Autodesk Inventor part; units mm, degrees
ref_plane "YZ Plane" through (0, 0, 0) normal (1, 0, 0) x (0, 1, 0)
ref_plane "XZ Plane" through (0, 0, 0) normal (0, 1, 0) x (-1, 0, 0)
ref_plane "XY Plane" through (0, 0, 0) normal (0, 0, 1) x (1, 0, 0)
sketch "Sketch1" plane through (0, 0, 0) normal (0, 0, 1) x (1, 0, 0)
  line L0 (-12.1708, 16.0073) -> (13.2292, 16.0073)
  line L1 (13.2292, 16.0073) -> (13.2292, -34.7927)
  line L2 (13.2292, -34.7927) -> (-12.1708, -34.7927)
  line L3 (-12.1708, -34.7927) -> (-12.1708, 16.0073)
  line L4 (11.9592, 14.7373) -> (-10.9008, 14.7373)
  line L5 (-10.9008, 14.7373) -> (-10.9008, -33.5227)
  line L6 (-10.9008, -33.5227) -> (11.9592, -33.5227)
  line L7 (11.9592, -33.5227) -> (11.9592, 14.7373)
  point P0 (0, 0)
  dimension "d0" = 25.4
  dimension "d1" = 50.8
  dimension "d2" = 1.27
extrude "Extrusion1" add sketch "Sketch1" along normal blind 76.2
sketch "Sketch2" plane through (-12.1708, 16.0073, 0) normal (0, 1, 0) x (1, 0, 0)
  circle A0 centre (12.7, -12.7) radius 1.7272
  line L0 (25.4, 0) -> (0, 0)
  line L1 (0, 0) -> (0, -76.2)
  point P0 (12.1708, 0)
  dimension "d5" = 3.4544
  dimension "d6" = 12.7
  dimension "d7" = 12.7
extrude "Extrusion2" cut sketch "Sketch2" against normal through all
pattern_linear "Rectangular Pattern1" count 8 spacing 25.4 along (0, 0, 1) of "Extrusion2"
sketch "Sketch3" plane through (13.2292, -34.7927, 0) normal (1, 0, 0) x (0, 0, -1)
  circle A0 centre (-38.1, 25.4) radius 14.2875
  line L0 (0, 0) -> (-76.2, 0)
  line L1 (-76.2, 0) -> (-76.2, 50.8)
  point P0 (0, 34.7927)
  dimension "d15" = 25.4
  dimension "d16" = 38.1
  dimension "d17" = 28.575
extrude "Extrusion3" cut sketch "Sketch3" against normal through all
equation "\"d3\" = d13"
equation "\"d10\" = d14"
equation "\"d13\" = 76.2"
equation "\"d14\" = d13"
properties part number "Test  Stock Rotation extender"
Input: part model. Units: mm. Frame: model coordinates. A direction names the side the tool comes from. Coordinates: 2 decimals unless noted, no trailing zeros. Order: outer loops, then holes, each group sorted by start corner. A loop starts at its lowest first (then second) coordinate and runs counter-clockwise, first axis right, second up. Notation, with made-up numbers: M -14.5,56.5 L 32.5,56.5 A12 ccw 32.5,60.5 Z; hole C 49,81 d11. An arc over 180 degrees is marked long. Write item = value, one per line. Start each with the question number.
(1) Section C-C on x = -2. Output: boundary loops of the cut face in (y, z).
(2) Section A-A on z = 12.7. Output: boundary loops of the cut face in (x, y).
(3) Section D-D on z = 38.1. Output: boundary loops of the cut face in (x, y), and give its area (3 significant figures).
(4) Pull-direction query (Z, two-part tool) for faces 3 (the flat face through (-10.901, 7, 38)), 4 (the cylindrical face through (0.3, -34.15, 10.99)), 5 (the flat face through (-12, -9, 0)), 6 (the cylindrical face through (12.603, -5.101, 24.472)); classes: released by +Z, released by -Z, zero draft, split by the parting line, or undercut.
(5) Section B-B on y = -28.5. Output: boundary loops of the cut face in (x, z).
(6) First-contact query: P1, Ø2, axis at x = 0.53, z = 12.7, coming from the +Y side. Flat tip, straight axial feed; report the tip coordinate or a pass-through.
(7) Line query: line 1 along X through (y, z) = (-33.95, 38.1); line 2 along Y through (x, z) = (-10.5, 13.5); line 3 along X through (y, z) = (-19.5, 17.5). Output: solid intervals per line, ascending. Write a range as [from, to].
(8) Reachability of faces 1 (the flat face through (4, -34.793, 38)), 2 (the flat face through (11.959, 6, 38)) from +Z, -Z, +X, -X, +Y, -Y: full face, straight path, thin tool, end or side. Return the list, or none.
Result set:
q1.outline = M -34.79,0 L -33.52,0 L -33.52,76.2 L -34.79,76.2 Z; M 14.74,0 L 16.01,0 L 16.01,76.2 L 14.74,76.2 Z
q2.outline = M -12.17,-34.79 L -1.2,-34.79 L -1.2,-33.52 L -10.9,-33.52 L -10.9,14.74 L -1.2,14.74 L -1.2,16.01 L -12.17,16.01 Z; M 2.26,-34.79 L 13.23,-34.79 L 13.23,16.01 L 2.26,16.01 L 2.26,14.74 L 11.96,14.74 L 11.96,-33.52 L 2.26,-33.52 Z
q3.outline = M -12.17,-34.79 L -1.2,-34.79 L -1.2,-33.52 L -10.9,-33.52 L -10.9,-23.68 L -12.17,-23.68 Z; M -12.17,4.89 L -10.9,4.89 L -10.9,14.74 L -1.2,14.74 L -1.2,16.01 L -12.17,16.01 Z; M 2.26,-34.79 L 13.23,-34.79 L 13.23,-23.68 L 11.96,-23.68 L 11.96,-33.52 L 2.26,-33.52 Z; M 2.26,14.74 L 11.96,14.74 L 11.96,4.89 L 13.23,4.89 L 13.23,16.01 L 2.26,16.01 Z
q3.area = 106 mm²
q4.face_3 = zero draft
q4.face_4 = undercut
q4.face_5 = released by -Z
q4.face_6 = undercut
q5.outline = M -12.17,0 L -10.9,0 L -10.9,76.2 L -12.17,76.2 Z; M 11.96,0 L 13.23,0 L 13.23,76.2 L 11.96,76.2 Z
q6.P1 = through
q7.line_1 = [-12.17, -1.2], [2.26, 13.23]
q7.line_2 = [-34.79, -33.52], [14.74, 16.01]
q7.line_3 = [-12.17, -10.9], [11.96, 13.23]
q8.face_1 = +Z, -Z, +X, -X, -Y
q8.face_2 = +Z, -Z
